Source: CAD feature listing. Evaluate the final solid. Frame: model axes, mm. Give positions to 0.01 mm unless a question says otherwise; leave off trailing zeros. Write each loop counter-clockwise with the first axis right and the second up, starting at its lowest first coordinate (ties: lowest second). Pieces come first, ordered by that corner, then holes. Notation, with made-up numbers: M 36.5,5.25 L 80.5,5.25 A17 ccw 80.5,13.25 Z; hole C 1,25.25 d10. An arc over 180 degrees is marked long. Use CSV: the item, a comma, the result in double quotes. Start each with the question number.
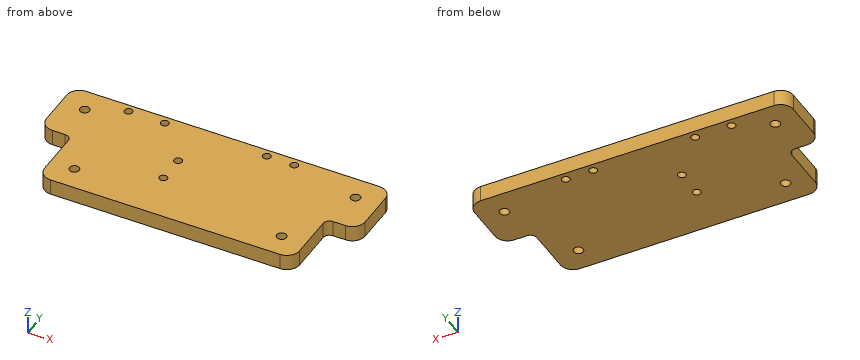
from build123d import *

# Parameters (mm, degrees)
SKETCH1_R           = 1.89865
SKETCH1_R_2         = 1.5875
BOSS_EXTRUDE1_DEPTH = 6.35
FILLET1_R           = 5.08
FILLET2_R           = 2.54


with BuildPart() as part:
    # Sketch1 → Boss-Extrude1 (new body)
    with BuildSketch(Plane.XY):
        Polygon((0, 50.8), (0, 25.4), (12.7, 25.4), (12.7, 0), (114.3, 0), (114.3, 25.4), (127, 25.4), (127, 50.8), align=None)
        with Locations((22.225, 9.525)):
            Circle(SKETCH1_R, mode=Mode.SUBTRACT)
        with Locations((52.324, 19.558)):
            Circle(SKETCH1_R_2, mode=Mode.SUBTRACT)
        with Locations((104.775, 9.525)):
            Circle(SKETCH1_R, mode=Mode.SUBTRACT)
        with Locations((52.324, 30.734)):
            Circle(SKETCH1_R_2, mode=Mode.SUBTRACT)
        with Locations((9.525, 41.275)):
            Circle(SKETCH1_R, mode=Mode.SUBTRACT)
        with Locations((23.622, 47.625)):
            Circle(SKETCH1_R_2, mode=Mode.SUBTRACT)
        with Locations((38.1, 47.625)):
            Circle(SKETCH1_R_2, mode=Mode.SUBTRACT)
        with Locations((78.74, 47.625)):
            Circle(SKETCH1_R_2, mode=Mode.SUBTRACT)
        with Locations((89.662, 47.625)):
            Circle(SKETCH1_R_2, mode=Mode.SUBTRACT)
        with Locations((117.475, 41.275)):
            Circle(SKETCH1_R, mode=Mode.SUBTRACT)
    extrude(amount=BOSS_EXTRUDE1_DEPTH)

    # Fillet1
    fillet1_edges = [part.edges().sort_by_distance(p)[0] for p in [
        (114.3, 0, 3.175),
        (12.7, 0, 3.175),
        (0, 25.4, 3.175),
        (0, 50.8, 3.175),
        (127, 50.8, 3.175),
        (127, 25.4, 3.175),
    ]]
    fillet(fillet1_edges, radius=FILLET1_R)

    # Fillet2
    fillet2_edges = [part.edges().sort_by_distance(p)[0] for p in [
        (12.7, 25.4, 3.175),
        (114.3, 25.4, 3.175),
    ]]
    fillet(fillet2_edges, radius=FILLET2_R)


solid = part.part
1. Line query: probe 1 along Y at (x, z) = (23, 1.5); probe 2 along Y at (x, z) = (105, 0.5); probe 3 along Y at (x, z) = (38.1, 2.25). Output: solid intervals per line, ascending.
2. Section B-B on z = 2.25. Give the number of separate pieces and of enclosed holes in the cut face, then the cut area to 3 significant figures.
3. Section C-C on y = 27.5. Return loops of the section in (x, z).
4. First-contact query: pin 1 (3.5 mm diameter, centred on x = 117.475, y = 41.275, fed in from +Z); pin 2 (2.5 mm diameter, centred on x = 8.5, z = 3, fed in from -Y); pin 3 (3 mm diameter, centred on y = 12, z = 4, fed in from -X). Flat tips, straight axial feed; report the tip coordinate or a pass-through.
5. Section A-A on x = 38.1. Return loops of the section in (y, z).
Resolved:
1,probe 1,"y = 0 to 7.79, 11.26 to 46.16, 49.09 to 50.8"
1,probe 2,"y = 0 to 7.64, 11.41 to 50.8"
1,probe 3,"y = 0 to 46.04, 49.21 to 50.8"
2,separate pieces,"1"
2,enclosed holes,"10"
2,area,"5,680 mm2"
3,outline,"M 0.97,0 L 126.03,0 L 126.03,6.35 L 0.97,6.35 Z"
4,pin 1,"passes through"
4,pin 2,"stops at y = 25.4"
4,pin 3,"stops at x = 12.7"
5,outline,"M 0,0 L 46.04,0 L 46.04,6.35 L 0,6.35 Z; M 49.21,0 L 50.8,0 L 50.8,6.35 L 49.21,6.35 Z"
